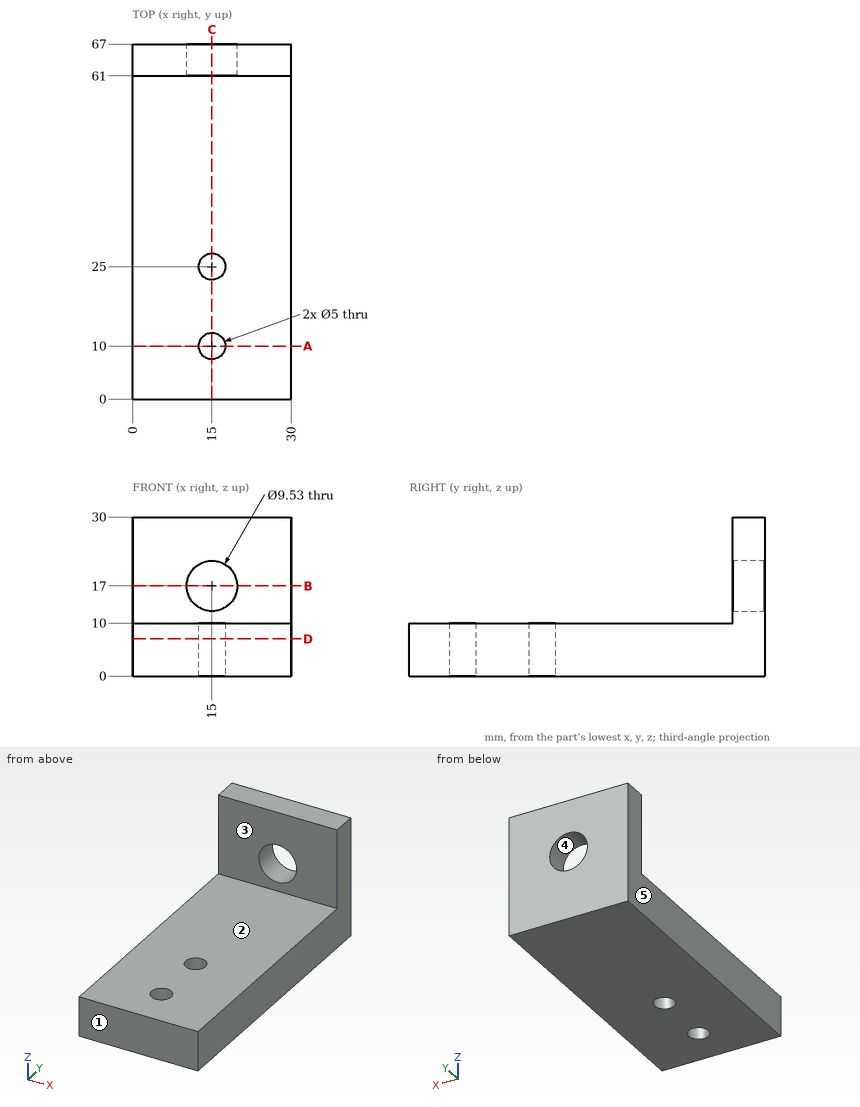
Design review of the part shown in the three views and the two pictorial views. Dimensions are in mm from the part's minimum x, y and z. A direction names the side the tool comes from. Give positions to 0.01 mm unless a question says otherwise; leave off trailing zeros. Write each loop counter-clockwise with the first axis right and the second up, starting at its lowest first coordinate (ties: lowest second). Pieces come first, ordered by that corner, then holes. Notation, with made-up numbers: M 60.5,78 L 88.5,78 A27 ccw 88.5,116 Z; hole C 36,-21 d3. An arc over 180 degrees is marked long. Return JSON: item names as keys, results as strings. Group by question number.
Item 1: Take a section at B-B (z = 17). Give the boundary of the cut face in (x, y) (3 decimals), plus the area to 3 significant figures.
Item 2: Wall thickness on line 1 along Y through (x, z) = (15, 4); line 2 along Z through (x, y) = (2.25, 51); line 3 along Y through (x, z) = (14.75, 28.5): over which ranges is each line inside the solid? List them lowest first.
Item 3: Clearance check with flat-ended pins moving along their axes: pin 1 Ø4 at (x, y) = (15, 25) entering from +Z; pin 2 Ø6 at (x, z) = (10.5, 20) entering from -Y; pin 3 Ø2 at (x, y) = (10.5, 43) entering from +Z. State where each tip first meets the part, or that it passes through.
Item 4: Take a section at A-A (y = 10). Give the boundary of the cut face in (x, z).
Item 5: The part is to be moulded in two halves that separate along X. For the marked faces 3, 4 and 5, say which applies: pulls with the +X half, pulls with the -X half, needs draft (parallel to the pull), parting line crosses it, or undercut.
Item 6: Take a section at C-C (x = 15). Give the boundary of the cut face in (y, z) (3 decimals), plus the area to 3 significant figures.
Item 7: Tool access review of the marked faces 1 and 2: name each direction out of +Z, -Z, +X, -X, +Y, -Y from which nothing blocks a thin tool from reaching the whole face with its end or side.
Item 8: Take a section at D-D (z = 7). Give the boundary of the cut face in (x, y).
Return value:
{
 "1": {"outline": "M 0,61 L 10.235,61 L 10.235,67 L 0,67 Z; M 19.765,61 L 30,61 L 30,67 L 19.765,67 Z", "area": "123 mm2"},
 "2": {"line 1": "y = 0 to 7.5, 12.5 to 22.5, 27.5 to 67", "line 2": "z = 0 to 10", "line 3": "y = 61 to 67"},
 "3": {"pin 1": "passes through", "pin 2": "stops at y = 61", "pin 3": "stops at z = 10"},
 "4": {"outline": "M 0,0 L 12.5,0 L 12.5,10 L 0,10 Z; M 17.5,0 L 30,0 L 30,10 L 17.5,10 Z"},
 "5": {"face 3": "needs draft", "face 4": "undercut", "face 5": "pulls with the -X half"},
 "6": {"outline": "M 0,0 L 7.5,0 L 7.5,10 L 0,10 Z; M 12.5,0 L 22.5,0 L 22.5,10 L 12.5,10 Z; M 27.5,0 L 67,0 L 67,12.235 L 61,12.235 L 61,10 L 27.5,10 Z; M 61,21.765 L 67,21.765 L 67,30 L 61,30 Z", "area": "633 mm2"},
 "7": {"face 1": "+Z, -Z, +X, -X, -Y", "face 2": "+Z, +X, -X, -Y"},
 "8": {"outline": "M 0,0 L 30,0 L 30,67 L 0,67 Z; hole C 15,10 d5; hole C 15,25 d5"}
}
